Can you work these out from the model? Positions are in its coordinate system, mm. A direction names the side the tool comes from. Round coordinates to 2 decimals unless told otherwise and drop trailing zeros. Order: outer loops, then holes, each group sorted by start corner. A loop starts at its lowest first (then second) coordinate and runs counter-clockwise, first axis right, second up.
from build123d import *

# Parameters (mm, degrees)
F0_W     = 20
F0_H     = 80
F1_DEPTH = 24
F0_W_2   = 30
F0_H_2   = 30
F2_DEPTH = 15
F3_DEPTH = 124
F4_R     = 15
F5_R     = 5
F6_D     = 10
F7_R     = 15
F8_DEPTH = 52


with BuildPart() as f1:
    # F0 (on Top) → F1 (new body)
    with BuildSketch(Plane.XY):
        Polygon((-50, -80), (50, -80), (50, -50), (80, -50), (80, 50), (50, 50), (50, 80), (-50, 80), (-50, 50), (-80, 50), (-80, -50), (-50, -50), align=None)
        with Locations((-30, 0)):
            Rectangle(F0_W, F0_H, mode=Mode.SUBTRACT)
        with Locations((30, 0)):
            Rectangle(F0_W, F0_H, mode=Mode.SUBTRACT)
    extrude(amount=F1_DEPTH)

    # F0 (on Top) → F2 (join)
    with BuildSketch(Plane.XY):
        with Locations((-65, -65)):
            Rectangle(F0_W_2, F0_H_2)
        with Locations((65, -65)):
            Rectangle(F0_W_2, F0_H_2)
        with Locations((65, 65)):
            Rectangle(F0_W_2, F0_H_2)
        with Locations((-65, 65)):
            Rectangle(F0_W_2, F0_H_2)
    extrude(amount=F2_DEPTH)

    # F0 (on Top) → F3 (join)
    with BuildSketch(Plane.XY):
        with Locations((-30, 0)):
            Rectangle(F0_W, F0_H)
        with Locations((30, 0)):
            Rectangle(F0_W, F0_H)
    extrude(amount=F3_DEPTH)

    # F4
    f4_edges = [f1.edges().sort_by_distance(p)[0] for p in [
        (-30, -40, 124),
        (30, -40, 124),
        (30, 40, 124),
        (-30, 40, 124),
        (-80, -80, 7.5),
        (80, -80, 7.5),
        (-80, 80, 7.5),
        (80, 80, 7.5),
    ]]
    fillet(f4_edges, radius=F4_R)

    # F5
    f5_edges = [f1.edges().sort_by_distance(p)[0] for p in [
        (50, 50, 19.5),
        (-50, 50, 19.5),
        (-50, -50, 19.5),
        (50, -50, 19.5),
    ]]
    fillet(f5_edges, radius=F5_R)

    # F6 (through all)
    with Locations(Plane(origin=(0, 0, 0), x_dir=(1, 0, 0), z_dir=(0, 0, -1))):
        with Locations((-65, 65), (-65, -65), (65, -65), (65, 65)):
            Hole(F6_D / 2)

    # F7 (on Right) → F8 (cut, symmetric)
    with BuildSketch(Plane.YZ):
        with Locations((0, 94)):
            Circle(F7_R)
    extrude(amount=F8_DEPTH, both=True, mode=Mode.SUBTRACT)


solid = f1.part
(1) If we mould it in two halves opening along Y, with no side actions, what happens to faces 1 (the face through (40, -1, 73)), 2 (the face through (68, 50, 19)), 3 (the face through (-68, -69, 8))? For each: pulls with the +Y half, pulls with the -Y half, needs draft (parallel to the pull), parting line crosses it, or undercut.
(2) I'm going to push flat-ended pins straight in: pin 1 Ø10 at (y, z) = (-24, 82) entering from +X; pin 2 Ø24 at (x, y) = (69.5, 64) entering from +Z; pin 3 Ø4 at (y, z) = (-10.5, 87) entering from -X; pin 4 Ø10 at (x, y) = (-16.5, -37.5) entering from +Z. Where does each tip first touch, or does it pass through?
(3) Please list where these lines run through material, in increasing order: probe 1 along Y at (x, z) = (-65, 9.25); probe 2 along X at (y, z) = (-26.5, 105).
(4) I want a section at B-B, the plane z = 94. List the corners of the cut face in (x, y) for me.
(5) On a 3-axis mill with a long thin cutter (end or side, diameter ignored), from which of +Z, -Z, +X, -X, +Y, -Y can I reach the whole of each face in a straight line? I mean faces 4 (the face through (-30, 40, 66)), 5 (the face through (61, -61, 15)), 6 (the face through (-67, 50, 19)), 7 (the face through (-51, -52, 20)), 8 (the face through (-30, -40, 66)). Say none if no direction works.
(6) I want a section at D-D, the plane z = 113. List the corners of the cut face in (x, y) for me.
(7) I want a section at A-A, the plane z = 30.5. List the corners of the cut face in (x, y) for me.
(8) I want a section at C-C, the plane y = 0. List the corners of the cut face in (x, z) for me.
Ans:
1. face 1: needs draft
1. face 2: pulls with the +Y half
1. face 3: undercut
2. pin 1: stops at x = 40
2. pin 2: stops at z = 15
2. pin 3: passes through
2. pin 4: stops at z = 121.05
3. probe 1: y = -80 to -70, -60 to 60, 70 to 80
3. probe 2: x = -40 to -20, 20 to 40
4. outline: (-40, -40) - (-20, -40) - (-20, -15) - (-40, -15) - close; (-40, 15) - (-20, 15) - (-20, 40) - (-40, 40) - close; (20, -40) - (40, -40) - (40, -15) - (20, -15) - close; (20, 15) - (40, 15) - (40, 40) - (20, 40) - close
5. face 4: +Z, +X, -X, +Y
5. face 5: +Z, +X, -Y
5. face 6: +Z, -X, +Y
5. face 7: +Z, -X, -Y
5. face 8: +Z, +X, -X, -Y
6. outline: (-40, -39.46) - (-20, -39.46) - (-20, 39.46) - (-40, 39.46) - close; (20, -39.46) - (40, -39.46) - (40, 39.46) - (20, 39.46) - close
7. outline: (-40, -40) - (-20, -40) - (-20, 40) - (-40, 40) - close; (20, -40) - (40, -40) - (40, 40) - (20, 40) - close
8. outline: (-80, 0) - (80, 0) - (80, 24) - (40, 24) - (40, 79) - (20, 79) - (20, 24) - (-20, 24) - (-20, 79) - (-40, 79) - (-40, 24) - (-80, 24) - close; (-40, 109) - (-20, 109) - (-20, 124) - (-40, 124) - close; (20, 109) - (40, 109) - (40, 124) - (20, 124) - close
